from build123d import *

# Parameters (mm, degrees)
SKETCH_1_W              = 40
SKETCH_1_H              = 75
EXTRUDE_1_DEPTH         = 20
SKETCH_2_W              = 36
SKETCH_2_H              = 71
CUT_EXTRUDE_1_DEPTH     = 18
CUT_EXTRUDE4_DEPTH      = 47.97073557
CUT_EXTRUDE4_DEPTH_BACK = 47.97073557
SKETCH1_R               = 1.5


with BuildPart() as part:
    # 스케치1 → 보스-돌출1 (new body)
    with BuildSketch(Plane(origin=(0, 0, 0), x_dir=(1, 0, 0), z_dir=(0, 1, 0))):
        Rectangle(SKETCH_1_W, SKETCH_1_H)
    extrude(amount=EXTRUDE_1_DEPTH)

    # 스케치2 → 컷-돌출1 (cut)
    with BuildSketch(Plane(origin=(0, 20, 0), x_dir=(1, 0, 0), z_dir=(0, 1, 0))):
        Rectangle(SKETCH_2_W, SKETCH_2_H)
    extrude(amount=-CUT_EXTRUDE_1_DEPTH, mode=Mode.SUBTRACT)

    # Sketch1 → Cut-Extrude4 (cut, two sides: drawn at the far end of the back side and taken through both)
    with BuildSketch(Plane(origin=(0, 0, 0), x_dir=(1, 0, 0), z_dir=(0, 1, 0)).offset(-CUT_EXTRUDE4_DEPTH_BACK)):
        with Locations(Location((-10, 0, 0), (0, 0, 270))):
            Circle(SKETCH1_R)
        with Locations(Location((10, 0, 0), (0, 0, 270))):
            Circle(SKETCH1_R)
    extrude(amount=CUT_EXTRUDE4_DEPTH + CUT_EXTRUDE4_DEPTH_BACK, mode=Mode.SUBTRACT)


solid = part.part
Source: CAD feature listing. Evaluate the final solid. Frame: model axes, mm. A direction names the side the tool comes from. Coordinates: 2 decimals unless noted, no trailing zeros. Loops run counter-clockwise (first coordinate to the right, second up) from the corner with the lowest first, then second, coordinate; pieces in that order, holes last. Notation, with made-up numbers: (48.25, -5) -> (93.25, -5) arc R14 cw to (93.25, 0) -> close; hole circle Ø1 at (65.25, 64.25). An arc over 180 degrees is marked (long way). Answer in a Markdown table with one row per item. Add a question column.
Q1. Ray query, line 1 along X through (y, z) = (1, 0); line 2 along Z through (x, y) = (-10, 0.7); line 3 along X through (y, z) = (7.75, 23). Return the intervals inside material, ascending.
Q2. Section A-A on x = 10. Return the cut outline in (y, z), and give its area (3 significant figures).
Q3. Pull-direction query (X, two-part tool) for faces 1 (the face through (0, 10, -37.5)), 2 (the face through (0, 2, 0)), 3 (the face through (-20, 10, 1)), 4 (the face through (-18, 11, 0)); classes: pulls with the +X half, pulls with the -X half, needs draft (parallel to the pull), parting line crosses it, or undercut.
Q4. Reachability of faces 5 (the face through (0, 11, 35.5)), 6 (the face through (20, 10, 1)) from +Z, -Z, +X, -X, +Y, -Y: full face, straight path, thin tool, end or side. Return the list, or none.
Q5. Section D-D on x = -16.5. Return the cut outline in (y, z).
Q6. Section B-B on y = 10.5. Return the cut outline in (x, z), and give its area (3 significant figures).
Q7. Section C-C on z = 0. Return the cut outline in (x, y), and give its area (3 significant figures).
Q8. Contact query for a flat-ended pin moving along its axis: pin 1 Ø18 at (x, z) = (-0.5, 0.5) entering from +Y. Output: stop coordinate, or through.
Computed values:
| question | item | result |
|---|---|---|
| 1 | line 1 | x = -20 to -11.5, -8.5 to 8.5, 11.5 to 20 |
| 1 | line 2 | z = -37.5 to -1.5, 1.5 to 37.5 |
| 1 | line 3 | x = -20 to -18, 18 to 20 |
| 2 | outline | (0, -37.5) -> (20, -37.5) -> (20, -35.5) -> (2, -35.5) -> (2, -1.5) -> (0, -1.5) -> close; (0, 1.5) -> (2, 1.5) -> (2, 35.5) -> (20, 35.5) -> (20, 37.5) -> (0, 37.5) -> close |
| 2 | area | 216 mm^2 |
| 3 | face 1 | needs draft |
| 3 | face 2 | undercut |
| 3 | face 3 | pulls with the -X half |
| 3 | face 4 | undercut |
| 4 | face 5 | +Y |
| 4 | face 6 | +Z, -Z, +X, +Y, -Y |
| 5 | outline | (0, -37.5) -> (20, -37.5) -> (20, -35.5) -> (2, -35.5) -> (2, 35.5) -> (20, 35.5) -> (20, 37.5) -> (0, 37.5) -> close |
| 6 | outline | (-20, -37.5) -> (20, -37.5) -> (20, 37.5) -> (-20, 37.5) -> close; hole (-18, -35.5) -> (18, -35.5) -> (18, 35.5) -> (-18, 35.5) -> close |
| 6 | area | 444 mm^2 |
| 7 | outline | (-20, 0) -> (-11.5, 0) -> (-11.5, 2) -> (-18, 2) -> (-18, 20) -> (-20, 20) -> close; (-8.5, 0) -> (8.5, 0) -> (8.5, 2) -> (-8.5, 2) -> close; (11.5, 0) -> (20, 0) -> (20, 20) -> (18, 20) -> (18, 2) -> (11.5, 2) -> close |
| 7 | area | 140 mm^2 |
| 8 | pin 1 | stops at y = 2 |
